from build123d import *

# Parameters (mm, degrees)
BASE_FLANGE1_DEPTH = 3
SKETCH23_R         = 1.65
CUT_EXTRUDE3_DEPTH = 3


# Sheet-metal steps are written as plain solids
with BuildPart() as part:
    # Sketch1 → Base-Flange1 (new body)
    with BuildSketch(Plane(origin=(0, 0, 0), x_dir=(1, 0, 0), z_dir=(0, 1, 0))):
        with BuildLine():
            Line((-63.892333426, 101.078420902), (-95.697333426, 5.100954406))
            ThreePointArc((-95.697333426, 5.100954406), (-95.212546513, 1.951017377), (-92.375, 0.5))
            Line((-92.375, 0.5), (92.375, 0.5))
            ThreePointArc((92.375, 0.5), (95.212546513, 1.951017377), (95.697333426, 5.100954406))
            Line((95.697333426, 5.100954406), (63.892333426, 101.078420902))
            ThreePointArc((63.892333426, 101.078420902), (62.618982623, 102.815013009), (60.57, 103.477466496))
            Line((60.57, 103.477466496), (-60.57, 103.477466496))
            ThreePointArc((-60.57, 103.477466496), (-62.618982623, 102.815013009), (-63.892333426, 101.078420902))
        make_face()
    extrude(amount=-BASE_FLANGE1_DEPTH)

    # Sketch23 → Cut-Extrude3 (cut)
    with BuildSketch(Plane.XZ.offset(3)):
        with Locations(Location((-82, -12.182416465, 0), (0, 0, 270))):
            Circle(SKETCH23_R)
        with Locations(Location((82, -12.182416465, 0), (0, 0, 270))):
            Circle(SKETCH23_R)
        with Locations(Location((58.757797989, -98.719801772, 0), (0, 0, 270))):
            Circle(SKETCH23_R)
        with Locations(Location((-59.392713729, -98.076633575, 0), (0, 0, 270))):
            Circle(SKETCH23_R)
    extrude(amount=-CUT_EXTRUDE3_DEPTH, mode=Mode.SUBTRACT)


solid = part.part
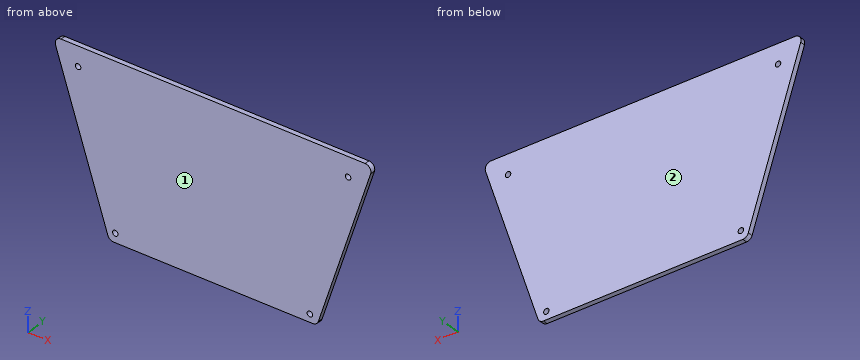
Part model, mm, in its own coordinate system. Face numbers are marked on the shaded views. Coordinates: 2 decimals unless noted, no trailing zeros. Loops run counter-clockwise (first coordinate to the right, second up) from the corner with the lowest first, then second, coordinate; pieces in that order, holes last. Notation, with made-up numbers: (-25.75, -24.75) -> (17.25, -24.75) arc R13 cw to (17.25, -19.75) -> close; hole circle Ø1 at (33, -27.5). An arc over 180 degrees is marked (long way). Use a Markdown table: item, result. Add a question column.
Item 1: Band-saw the part on A-A on y = -2. Write the cut outline in (x, z) (3 decimals), plus the area to 3 significant figures.
Item 2: Probe probe 1 along X at (y, z) = (-0.6, -11); probe 2 along X at (y, z) = (-1.95, -13.5); probe 3 along X at (y, z) = (-2.2, -18). List the from-to ranges inside material, lowest first.
Item 3: Pull direction Y, two halves, no side cores. Call the marked faces 1 and 2: +Y half, -Y half, draft (parallel to the pull), parting line (faces both ways), or undercut.
Item 4: Band-saw the part on B-B on z = -51.5. Write the cut outline in (x, y).
Item 5: Band-saw the part on C-C on z = -92. Write the cut outline in (x, y), plus the area to 3 significant figures.
Geometry says:
| question | item | result |
|---|---|---|
| 1 | outline | (-95.697, -5.101) -> (-63.892, -101.078) arc R3.5 ccw to (-60.57, -103.477) -> (60.57, -103.477) arc R3.5 ccw to (63.892, -101.078) -> (95.697, -5.101) arc R3.5 ccw to (92.375, -0.5) -> (-92.375, -0.5) arc R3.5 ccw to start; hole circle Ø3.3 at (-82, -12.182); hole circle Ø3.3 at (-59.393, -98.077); hole circle Ø3.3 at (58.758, -98.72); hole circle Ø3.3 at (82, -12.182) |
| 1 | area | 16,500 mm² |
| 2 | probe 1 | -93.74 to -83.15, -80.85 to 80.85, 83.15 to 93.74 |
| 2 | probe 2 | -92.91 to -82.99, -81.01 to 81.01, 82.99 to 92.91 |
| 2 | probe 3 | -91.42 to 91.42 |
| 3 | face 1 | -Y half |
| 3 | face 2 | +Y half |
| 4 | outline | (-80.32, -3) -> (80.32, -3) -> (80.32, 0) -> (-80.32, 0) -> close |
| 5 | outline | (-66.9, -3) -> (66.9, -3) -> (66.9, 0) -> (-66.9, 0) -> close |
| 5 | area | 401 mm² |
